The listing builds one solid part. Answer for the finished solid, in the listing's coordinates (mm). Face numbers are marked on the shaded views. A direction names the side the tool comes from. Round coordinates to 2 decimals unless told otherwise and drop trailing zeros. Loops run counter-clockwise (first coordinate to the right, second up) from the corner with the lowest first, then second, coordinate; pieces in that order, holes last. Notation, with made-up numbers: (82.5, 20) - (103.5, 20) arc R10 cw to (103.5, 28) - close; hole circle Ø4 at (-15, 32.5). An arc over 180 degrees is marked (long way). One line per item, written item: value.
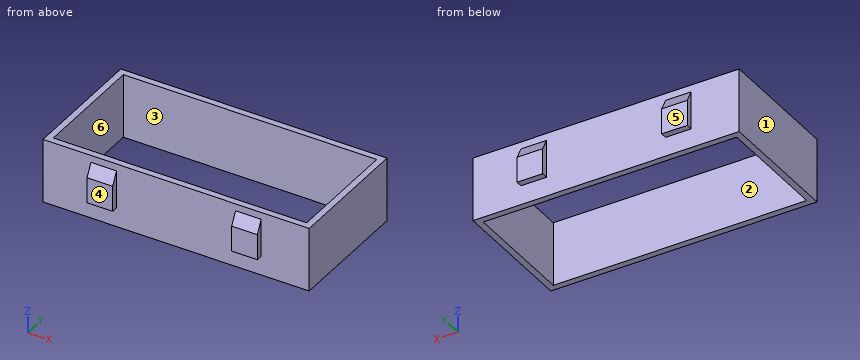
```python
from build123d import *

# Parameters (mm, degrees)
SKETCH1_W           = 41.6
SKETCH1_H           = 20
SKETCH1_W_2         = 39.6
SKETCH1_H_2         = 18
BOSS_EXTRUDE2_DEPTH = 10
SKETCH2_W           = 4
SKETCH2_H           = 10
BOSS_EXTRUDE3_DEPTH = 1
SKETCH3_W           = 3
SKETCH3_H           = 1
CUT_EXTRUDE1_DEPTH  = 27
SKETCH4_W           = 4
SKETCH4_H           = 10
BOSS_EXTRUDE4_DEPTH = 1
SKETCH5_W           = 3
SKETCH5_H           = 1
CUT_EXTRUDE2_DEPTH  = 27


with BuildPart() as part:
    # Sketch1 → Boss-Extrude2 (new body)
    with BuildSketch(Plane.XY):
        Rectangle(SKETCH1_W, SKETCH1_H)
        Rectangle(SKETCH1_W_2, SKETCH1_H_2, mode=Mode.SUBTRACT)
    extrude(amount=BOSS_EXTRUDE2_DEPTH)

    # Sketch2 → Boss-Extrude3 (add)
    with BuildSketch(Plane.XZ.offset(10)):
        with Locations((-11.3, 5)):
            Rectangle(SKETCH2_W, SKETCH2_H)
        with Locations((11.3, 5)):
            Rectangle(SKETCH2_W, SKETCH2_H)
    extrude(amount=BOSS_EXTRUDE3_DEPTH)

    # Sketch3 → Cut-Extrude1 (cut)
    with BuildSketch(Plane.ZY.offset(13.3)):
        Polygon((8.900149248, -10), (7, -11), (10, -11), (10, -10), align=None)
        with Locations((1.5, -10.5)):
            Rectangle(SKETCH3_W, SKETCH3_H)
    extrude(amount=-CUT_EXTRUDE1_DEPTH, mode=Mode.SUBTRACT)

    # Sketch4 → Boss-Extrude4 (add)
    with BuildSketch(Plane(origin=(0, 10, 0), x_dir=(1, 0, 0), z_dir=(0, 1, 0))):
        with Locations((11.3, -5)):
            Rectangle(SKETCH4_W, SKETCH4_H)
        with Locations((-11.3, -5)):
            Rectangle(SKETCH4_W, SKETCH4_H)
    extrude(amount=BOSS_EXTRUDE4_DEPTH)

    # Sketch5 → Cut-Extrude2 (cut)
    with BuildSketch(Plane(origin=(13.3, 0, 0), x_dir=(0, 0, -1), z_dir=(1, 0, 0))):
        Polygon((-7, 11), (-10, 11), (-10, 10), (-8.900149248, 10), align=None)
        with Locations((-1.5, 10.5)):
            Rectangle(SKETCH5_W, SKETCH5_H)
    extrude(amount=-CUT_EXTRUDE2_DEPTH, mode=Mode.SUBTRACT)


solid = part.part
```
1) For the marked faces 5 and 6, determine the directions among +Z, -Z, +X, -X, +Y, -Y from which every point of the face is accessible in a straight line to the end or side of a thin tool.
Final values:
face 5: +Z, -Z, +X, -X, +Y
face 6: +Z, -Z
2) Consider L1, parallel to X at y = -5.5, z = 9; L2, parallel to Y at x = -14.5, z = 2; L3, parallel to Y at x = -11, z = 4. Determine where each line is inside the solid, lowest interval first.
Final values:
L1: -20.8 to -19.8, 19.8 to 20.8
L2: -10 to -9, 9 to 10
L3: -11 to -9, 9 to 11
3) A cutting plane is placed at B-B on x = -3.5. Give the vertices of the cut face in (y, z).
Final values:
outline: (-10, 0) - (-9, 0) - (-9, 10) - (-10, 10) - close; (9, 0) - (10, 0) - (10, 10) - (9, 10) - close
4) For a pull along Y with two mould halves and no side action, classify the marked faces 1, 2, 3 and 4 as released by +Y, released by -Y, zero draft, split by the parting line, or undercut.
Final values:
face 1: zero draft
face 2: undercut
face 3: undercut
face 4: released by -Y
5) Each of these flat-tipped pins is pushed along its axis until it touches: pin 1 Ø0.5 at (x, y) = (11.5, -10.5) entering from -Z; pin 2 Ø3 at (x, z) = (9, 7) entering from -Y; pin 3 Ø0.5 at (y, z) = (10.5, 6) entering from +X; pin 4 Ø5 at (x, y) = (15, -1) entering from -Z. Where does it stop, or does it pass through?
Final values:
pin 1: z = 3
pin 2: y = -11
pin 3: x = 13.3
pin 4: through
6) A cutting plane is placed at C-C on z = 1.5. Give the vertices of the cut face in (x, y).
Final values:
outline: (-20.8, -10) - (20.8, -10) - (20.8, 10) - (-20.8, 10) - close; hole (-19.8, -9) - (19.8, -9) - (19.8, 9) - (-19.8, 9) - close
7) A cutting plane is placed at A-A on y = -6.5. Give the vertices of the cut face in (x, z).
Final values:
outline: (-20.8, 0) - (-19.8, 0) - (-19.8, 10) - (-20.8, 10) - close; (19.8, 0) - (20.8, 0) - (20.8, 10) - (19.8, 10) - close
8) A cutting plane is placed at D-D on x = -11.5. Give the vertices of the cut face in (y, z), and give its area (3 significant figures).
Final values:
outline: (-11, 3) - (-10, 3) - (-10, 0) - (-9, 0) - (-9, 10) - (-10, 10) - (-10, 8.9) - (-11, 7) - close; (9, 0) - (10, 0) - (10, 3) - (11, 3) - (11, 7) - (10, 8.9) - (10, 10) - (9, 10) - close
area: 29.9 mm2
